Can you work these out from the model? Positions are in its coordinate system, mm. Give positions to 0.01 mm unless a question says otherwise; leave off trailing zeros. Write each loop counter-clockwise with the first axis right and the second up, starting at its lowest first coordinate (ties: lowest second). Pieces come first, ordered by that corner, then holes.
1. Suppose I cut it at A-A (x = 0). Please give me the cut outline in (y, z).
2. Suppose I cut it at C-C (z = 0). Please give me the cut outline in (x, y), and give its area (3 significant figures).
3. I'm going to push flat-ended pins straight in: pin 1 (2 mm diameter, centred on x = 8, y = 2.5, fed in from -Z); pin 2 (8.5 mm diameter, centred on x = 0, z = 47.5, fed in from -Y); pin 3 (1 mm diameter, centred on x = 16.5, y = 2.5, fed in from +Z); pin 4 (1.5 mm diameter, centred on x = -35.5, z = -43, fed in from -Y). Where does each tip first touch, or does it pass through?
4. Suppose I cut it at B-B (y = 0.9). Give the number of separate pieces and of enclosed holes in the cut face, and give its area (3 significant figures).
5. Suppose I cut it at D-D (z = 29). Please give me the cut outline in (x, y).
6. If I drill on probe 1 along X at (y, z) = (3.05, 29.5); probe 2 along X at (y, z) = (0.6, -42.5); probe 3 along Z at (x, y) = (-20.5, 3.7), over which ranges is the centre line in solid material (lowest first)?
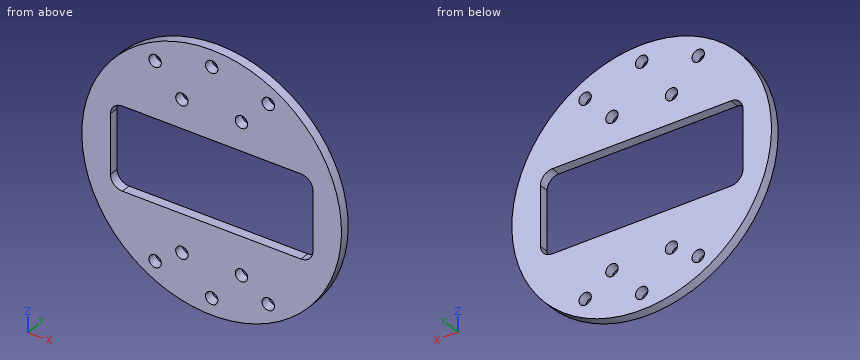
```python
from build123d import *

# Parameters (mm, degrees)
SKETCH_1_R               = 54.5
EXTRUDE_1_DEPTH          = 4
SKETCH_2_W               = 85
SKETCH_2_H               = 35
CUT_EXTRUDE_1_DEPTH      = 4
FILLET_1_R               = 5
SKETCH_3_R               = 2.6
CUT_EXTRUDE_2_DEPTH      = 10
PATTERN_CIRCULAR_1_COUNT = 2
SKETCH_4_R               = 2.6
CUT_EXTRUDE_3_DEPTH      = 10
SKETCH_5_R               = 2.6
CUT_EXTRUDE_4_DEPTH      = 100


with BuildPart() as part:
    # 草图1 → 凸台-拉伸1 (new body)
    with BuildSketch(Plane(origin=(0, 0, 0), x_dir=(1, 0, 0), z_dir=(0, 1, 0))):
        with Locations(Location((0, 0, 0), (0, 0, 270))):
            Circle(SKETCH_1_R)
    extrude(amount=EXTRUDE_1_DEPTH)

    # 草图2 → 切除-拉伸1 (cut)
    with BuildSketch(Plane(origin=(0, 4, 0), x_dir=(1, 0, 0), z_dir=(0, 1, 0))):
        Rectangle(SKETCH_2_W, SKETCH_2_H)
    extrude(amount=-CUT_EXTRUDE_1_DEPTH, mode=Mode.SUBTRACT)

    # 圆角1
    fillet_1_edges = [part.edges().sort_by_distance(p)[0] for p in [
        (42.5, 2, -17.5),
        (42.5, 2, 17.5),
        (-42.5, 2, 17.5),
        (-42.5, 2, -17.5),
    ]]
    fillet(fillet_1_edges, radius=FILLET_1_R)

    # 草图3 → 切除-拉伸2 (cut)
    with BuildSketch(Plane.XZ):
        with Locations(Location((-23.75, 41.13620668, 0), (0, 0, 270))):
            Circle(SKETCH_3_R)
        with Locations(Location((23.75, 41.13620668, 0), (0, 0, 270))):
            Circle(SKETCH_3_R)
        with Locations(Location((0, 47.5, 0), (0, 0, 270))):
            Circle(SKETCH_3_R)
    cut_extrude_2 = extrude(amount=-CUT_EXTRUDE_2_DEPTH, mode=Mode.SUBTRACT)

    # 阵列(圆周)1: 切除-拉伸2 ×2 about axis
    pattern_circular_1_axis = Axis((0, 0, 0), (0, 1, 0))
    for i in range(1, PATTERN_CIRCULAR_1_COUNT):
        add(cut_extrude_2.rotate(pattern_circular_1_axis, i * 360 / PATTERN_CIRCULAR_1_COUNT), mode=Mode.SUBTRACT)

    # 草图4 → 切除-拉伸3 (cut)
    with BuildSketch(Plane.XZ):
        with Locations(Location((-12.5, 29.5, 0), (0, 0, 270))):
            Circle(SKETCH_4_R)
        with Locations(Location((12.5, 29.5, 0), (0, 0, 270))):
            Circle(SKETCH_4_R)
    extrude(amount=-CUT_EXTRUDE_3_DEPTH, mode=Mode.SUBTRACT)

    # 草图5 → 切除-拉伸4 (cut)
    with BuildSketch(Plane.XZ):
        with Locations(Location((-12.5, -33.5, 0), (0, 0, 270))):
            Circle(SKETCH_5_R)
        with Locations(Location((12.5, -33.5, 0), (0, 0, 270))):
            Circle(SKETCH_5_R)
    extrude(amount=-CUT_EXTRUDE_4_DEPTH, mode=Mode.SUBTRACT)


solid = part.part
```
Checks:
1. outline: (0, -54.5) - (4, -54.5) - (4, -50.1) - (0, -50.1) - close; (0, -44.9) - (4, -44.9) - (4, -17.5) - (0, -17.5) - close; (0, 17.5) - (4, 17.5) - (4, 44.9) - (0, 44.9) - close; (0, 50.1) - (4, 50.1) - (4, 54.5) - (0, 54.5) - close
2. outline: (-54.5, 0) - (-42.5, 0) - (-42.5, 4) - (-54.5, 4) - close; (42.5, 0) - (54.5, 0) - (54.5, 4) - (42.5, 4) - close
2. area: 96.0 mm2
3. pin 1: stops at z = -54.05
3. pin 2: stops at y = 0
3. pin 3: stops at z = 52.1
3. pin 4: passes through
4. separate pieces: 1
4. enclosed holes: 11
4. area: 6,170 mm2
5. outline: (-46.14, 0) - (-15.05, 0) - (-15.05, 4) - (-46.14, 4) - close; (-9.95, 0) - (9.95, 0) - (9.95, 4) - (-9.95, 4) - close; (15.05, 0) - (46.14, 0) - (46.14, 4) - (15.05, 4) - close
6. probe 1: x = -45.83 to -15.1, -9.9 to 9.9, 15.1 to 45.83
6. probe 2: x = -34.12 to -25.96, -21.54 to 21.54, 25.96 to 34.12
6. probe 3: z = -50.5 to -17.5, 17.5 to 50.5
